The model under review builds one solid part; all positions refer to its coordinate system, in mm. A direction names the side the tool comes from. Give positions to 0.01 mm unless a question says otherwise; leave off trailing zeros. Order: outer loops, then holes, each group sorted by start corner. A loop starts at its lowest first (then second) coordinate and runs counter-clockwise, first axis right, second up. Notation, with made-up numbers: (33, -27.5) - (73, -27.5) arc R25 ccw to (73, -9.5) - close; hole circle Ø6 at (36.5, -20.5). An arc over 180 degrees is marked (long way). Answer as CSV lines item,"result". Start each with the question number.
Autodesk Inventor part; units mm, degrees
ref_plane "YZ Plane" through (0, 0, 0) normal (1, 0, 0) x (0, 1, 0)
ref_plane "XZ Plane" through (0, 0, 0) normal (0, 1, 0) x (-1, 0, 0)
ref_plane "XY Plane" through (0, 0, 0) normal (0, 0, 1) x (1, 0, 0)
sketch "Boceto1" plane through (0, 0, 0) normal (0, 0, 1) x (1, 0, 0)
  line L0 (-20, 20) -> (20, 20)
  line L1 (20, 20) -> (20, -20)
  line L2 (20, -20) -> (-20, -20)
  line L3 (-20, -20) -> (-20, 20)
  line L4 (-20, 20) -> (20, -20) construction
  line L5 (-16, 16) -> (16, 16)
  line L6 (16, 16) -> (16, -16)
  line L7 (16, -16) -> (-16, -16)
  line L8 (-16, -16) -> (-16, 16)
  line L9 (-16, 0) -> (-20, 0) construction
  line L10 (0, 16) -> (0, 20) construction
  line L11 (16, 0) -> (20, 0) construction
  line L12 (0, -16) -> (0, -20) construction
  line L13 (-16, 16) -> (-16, 20)
  line L14 (16, -16) -> (20, -16)
  point P0 (0, 0)
  point P1 (0, 0)
  dimension "d0" = 40
  dimension "d1" = 4
  dimension "d4" = 40
extrude "Extrusión1" add sketch "Boceto1" along normal blind 1012 contours L0 L13 L8 L7 L14 L1 L2 L3
properties part number "C_358_40_2"
Item 1: Take a section at A-A on z = 91.5. Write out the cut boundary in (x, y).
Item 2: For line 1 along X through (y, z) = (-14, 413), list the stretches that pass through material, from the lowest coordinate up.
Item 3: Clearance check with flat-ended pins moving along their axes: pin 1 (18 mm diameter, centred on x = 10, z = 463.5, fed in from +Y); pin 2 (1.5 mm diameter, centred on y = 7.5, z = 230, fed in from +X). State where each tip first meets the part, or that it passes through.
Item 4: Take a section at B-B on x = -2. Write out the cut boundary in (y, z).
Item 5: Machinability: for faces 1 (the face through (-9, -16.2, 0)), 2 (the face through (-16, 2, 499)), which of the approach directions +Z, -Z, +X, -X, +Y, -Y give a long, thin tool a straight path to every point of the face, cutting with its end or side? Answer none if there is none.
Data:
1,outline,"(-20, -20) - (20, -20) - (20, -16) - (-16, -16) - (-16, 20) - (-20, 20) - close"
2,line 1,"x = -20 to -16"
3,pin 1,"stops at y = -16"
3,pin 2,"stops at x = -16"
4,outline,"(-20, 0) - (-16, 0) - (-16, 1012) - (-20, 1012) - close"
5,face 1,"-Z, +X, -X, +Y, -Y"
5,face 2,"+Z, -Z, +X, +Y"
